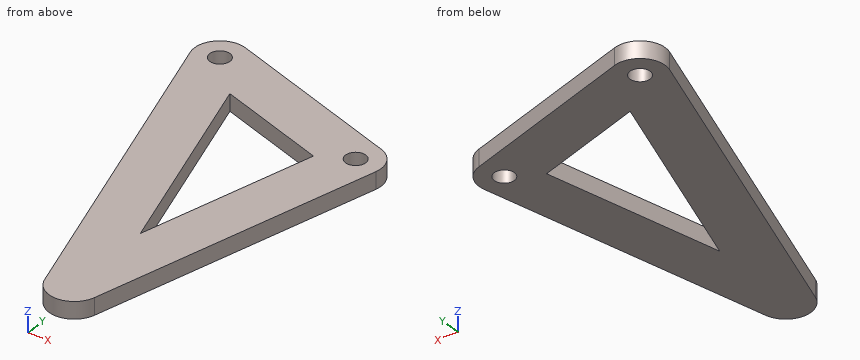
from build123d import *

# Parameters (mm, degrees)
BOSS_EXTRU_1_DEPTH           = 5
ENL_V_MAT_EXTRU_1_DEPTH      = 189.858435052
ENL_V_MAT_EXTRU_1_DEPTH_BACK = 189.858435052
ESQUISSE2_R                  = 3


with BuildPart() as part:
    # Esquisse1 → Boss.-Extru.1 (new body)
    with BuildSketch(Plane.XY):
        with BuildLine():
            Line((-111.688798728, -44.532571199), (-77.044116728, -146.825024533))
            ThreePointArc((-77.044116728, -146.825024533), (-69.528491269, -151.907819965), (-62.615784867, -146.03126267))
            Line((-62.615784867, -146.03126267), (-43.700257251, -60.088241923))
            ThreePointArc((-43.700257251, -60.088241923), (-44.549891694, -54.691461284), (-48.835290369, -51.302880733))
            Line((-48.835290369, -51.302880733), (-102.395499985, -34.953448145))
            ThreePointArc((-102.395499985, -34.953448145), (-109.968158579, -36.904307457), (-111.688798728, -44.532571199))
        make_face()
        Polygon((-59.838234907, -63.627479624), (-71.476166828, -116.504620821), (-92.791588673, -53.5683585), align=None, mode=Mode.SUBTRACT)
    extrude(amount=-BOSS_EXTRU_1_DEPTH)

    # Esquisse2 → Enlèv. mat.-Extru.1 (cut, two sides: drawn at the far end of the back side and taken through both)
    with BuildSketch(Plane.XY.offset(-ENL_V_MAT_EXTRU_1_DEPTH_BACK)):
        with Locations((-51.024946519, -58.476123092)):
            Circle(ESQUISSE2_R)
        with Locations((-104.585156135, -42.126690504)):
            Circle(ESQUISSE2_R)
    extrude(amount=ENL_V_MAT_EXTRU_1_DEPTH + ENL_V_MAT_EXTRU_1_DEPTH_BACK, mode=Mode.SUBTRACT)


solid = part.part
Model file for the job. Use its own axes, mm. Give positions to 0.01 mm unless a question says otherwise; leave off trailing zeros. Order: outer loops, then holes, each group sorted by start corner. A loop starts at its lowest first (then second) coordinate and runs counter-clockwise, first axis right, second up. Notation, with made-up numbers: M 21.5,-4 L 34.5,-4 A20 cw 34.5,18 Z; hole C 89,72 d5. An arc over 180 degrees is marked long. Put each result on its own line as item: value. Start each with the question number.
(1) Band-saw the part on B-B on y = -81. Give the cut face in (x, z).
(2) Band-saw the part on D-D on y = -141. Give the cut face in (x, z).
(3) Drill centre lines: L1, parallel to X at y = -91.5, z = -3.2; L2, parallel to X at y = -90, z = -1.4; L3, parallel to X at y = -136, z = -3.6. Where is each one in solid material? Low to high. Write a range as [from, to].
(4) Band-saw the part on A-A on x = -105.5. Give the cut face in (y, z).
(5) Pin check, flat tip, straight feed: pin 1 Ø3 at (y, z) = (-88, -3) entering from -X. Stop position of the tip, or through.
(6) Band-saw the part on C-C on z = -3.95. Give the cut face in (x, y).
Results below:
1. outline: M -99.34,-5 L -83.5,-5 L -83.5,0 L -99.34,0 Z; M -63.66,-5 L -48.3,-5 L -48.3,0 L -63.66,0 Z
2. outline: M -79.02,-5 L -61.51,-5 L -61.51,0 L -79.02,0 Z
3. L1: x = [-95.78, -79.94], [-65.97, -50.61]
3. L2: x = [-96.29, -80.45], [-65.64, -50.28]
3. L3: x = [-80.71, -60.41]
4. outline: M -62.81,-5 L -44.98,-5 L -44.98,0 L -62.81,0 Z; M -39.27,-5 L -34.68,-5 L -34.68,0 L -39.27,0 Z
5. pin 1: stops at x = -97.48
6. outline: M -111.69,-44.53 L -77.04,-146.83 A7.5 ccw -62.62,-146.03 L -43.7,-60.09 A7.5 ccw -48.84,-51.3 L -102.4,-34.95 A7.5 ccw Z; hole C -104.59,-42.13 d6; hole M -92.79,-53.57 L -71.48,-116.5 L -59.84,-63.63 Z; hole C -51.02,-58.48 d6
